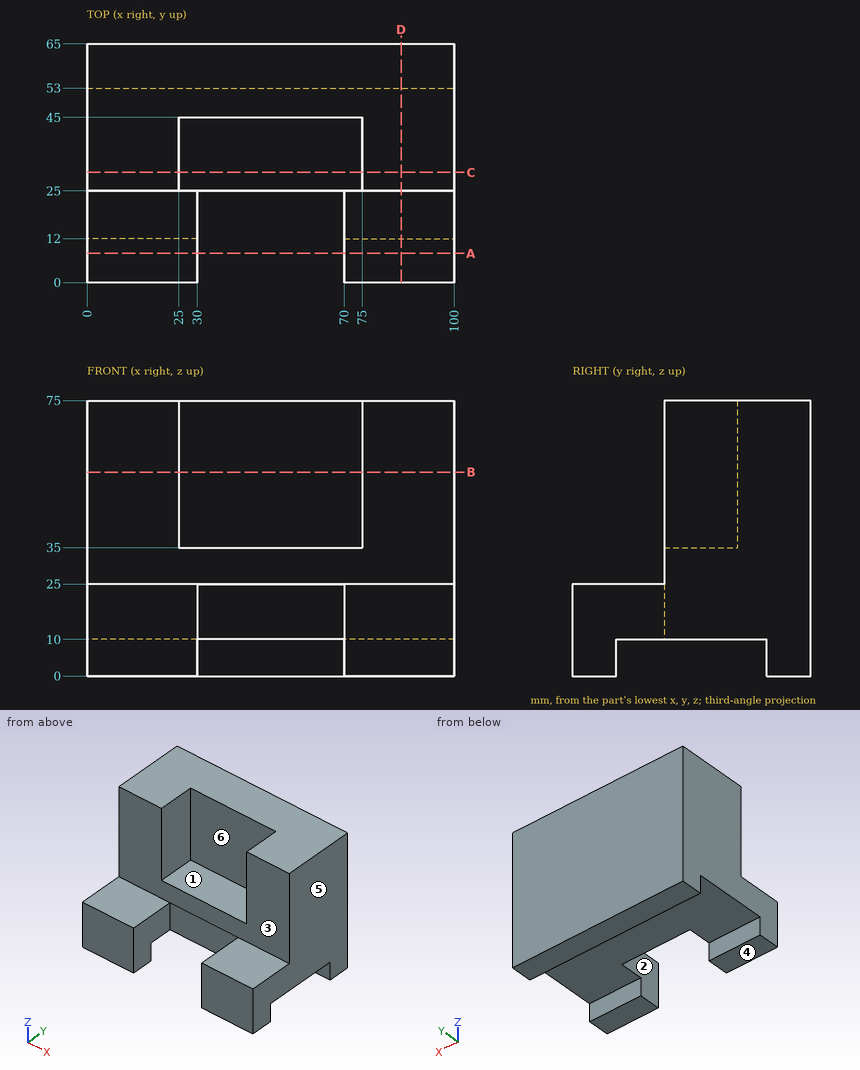
The drawing under review shows one solid part. Ordinate dimensions are in mm from its lowest x, y, z. A direction names the side the tool comes from. Coordinates: 2 decimals unless noted, no trailing zeros. Write each loop counter-clockwise with the first axis right and the second up, starting at its lowest first coordinate (ties: lowest second). Pieces come first, ordered by that corner, then holes. Notation, with made-up numbers: M -13,-6 L 36,-6 A16 cw 36,11 Z; hole C -39,76 d5. An arc over 180 degrees is marked long. Answer as a JSON object with one key per item and string values.
Item 1: Add section A-A, the plane y = 8. Give the boundary of the cut face in (x, z), and give its area (3 significant figures).
Outcome:
{"outline": "M 0,0 L 30,0 L 30,25 L 0,25 Z; M 70,0 L 100,0 L 100,25 L 70,25 Z", "area": "1,500 mm²"}
Item 2: Wall thickness on probe 1 along X at (y, z) = (39, 47); probe 2 along Y at (x, z) = (84.5, 8); probe 3 along Z at (x, y) = (28.5, 52.5): over which ranges is each line inside the solid? List them lowest first.
Outcome:
{"probe 1": "0 to 25, 75 to 100", "probe 2": "0 to 12, 53 to 65", "probe 3": "10 to 75"}
Item 3: Draft analysis for pull direction X (two halves, no side actions). For the marked faces 4, 5 and 6, state which applies: pulls with the +X half, pulls with the -X half, needs draft (parallel to the pull), parting line crosses it, or undercut.
Outcome:
{"face 4": "needs draft", "face 5": "pulls with the +X half", "face 6": "undercut"}
Item 4: Add section B-B, the plane z = 55.5. Give the boundary of the cut face in (x, y), and give its area (3 significant figures).
Outcome:
{"outline": "M 0,25 L 25,25 L 25,45 L 75,45 L 75,25 L 100,25 L 100,65 L 0,65 Z", "area": "3,000 mm²"}
Item 5: Insertion check: pin 1 Ø8 at (x, z) = (36.5, 38) entering from -Y; pin 2 Ø20 at (x, y) = (79.5, 12) entering from +Z; pin 3 Ø1.5 at (x, z) = (40.5, 42) entering from -Y. Each pin has a flat end and moves straight along its axis. Give the tip position at first contact, or say it passes through.
Outcome:
{"pin 1": "y = 25", "pin 2": "z = 25", "pin 3": "y = 45"}
Item 6: Machinability: for the marked faces 1, 2 and 3, which of the approach directions +Z, -Z, +X, -X, +Y, -Y give a long, thin tool a straight path to every point of the face, cutting with its end or side? Answer none if there is none.
Outcome:
{"face 1": "+Z, -Y", "face 2": "+Z, -Z, -Y", "face 3": "+Z, +X, -X, -Y"}
Item 7: Add section D-D, the plane x = 85.5. Give the boundary of the cut face in (y, z), and give its area (4 significant figures).
Outcome:
{"outline": "M 0,0 L 12,0 L 12,10 L 53,10 L 53,0 L 65,0 L 65,75 L 25,75 L 25,25 L 0,25 Z", "area": "3,215 mm²"}
Item 8: Add section C-C, the plane y = 30. Give the boundary of the cut face in (x, z).
Outcome:
{"outline": "M 0,10 L 100,10 L 100,75 L 75,75 L 75,35 L 25,35 L 25,75 L 0,75 Z"}
